Source: CAD feature listing. Evaluate the final solid. Frame: model axes, mm. A direction names the side the tool comes from. Give positions to 0.01 mm unless a question says otherwise; leave off trailing zeros. Loops run counter-clockwise (first coordinate to the right, second up) from the corner with the lowest first, then second, coordinate; pieces in that order, holes last. Notation, with made-up numbers: M 28,75.25 L 84,75.25 A30 ccw 84,110.25 Z; hole C -6.75,59 d11. An arc over 180 degrees is marked long. Write item = value, one per line.
from build123d import *

# Parameters (mm, degrees)
F1_DEPTH = 10
F2_R     = 1
F3_R     = 3
F4_R     = 0.33333


with BuildPart() as f1:
    # F0 (on Front) → F1 (new body)
    with BuildSketch(Plane.XZ):
        with BuildLine():
            Line((0, 0), (3.6, 0))
            Line((3.6, 0), (3.6, 3))
            Line((3.6, 3), (1.8, 3))
            Line((1.8, 3), (1.8, 11.7))
            Line((1.8, 11.7), (5.8, 11.7))
            Line((5.8, 11.7), (5.8, 8.7))
            Line((5.8, 8.7), (6.6518087818, 8.6985993288))
            ThreePointArc((6.6518087818, 8.6985993288), (7.4284566976, 8.3757785113), (7.75, 7.598600816))
            Line((7.75, 7.598600816), (9.25, 7.598600816))
            Line((9.25, 7.598600816), (7, 13.5))
            Line((7, 13.5), (0, 13.5))
            Line((0, 13.5), (0, 0))
        make_face()
        with BuildLine():
            ThreePointArc((6.4457045279, 5.2862485499), (8.0654097754, 6.1785827272), (9.25, 7.598600816))
            Line((9.25, 7.598600816), (7.75, 7.598600816))
            ThreePointArc((7.75, 7.598600816), (7.4278174593, 6.8207833567), (6.65, 6.498600816))
            Line((6.65, 6.498600816), (5.8, 6.498600816))
            Line((5.8, 6.498600816), (5.8, 5.2862485499))
            Line((5.8, 5.2862485499), (6.4457045279, 5.2862485499))
        make_face()
    extrude(amount=F1_DEPTH)

    # F2
    f2_edges = [f1.edges().sort_by_distance(p)[0] for p in [
        (0, -5, 13.5),
        (7, -5, 13.5),
        (6.445705, -5, 5.286249),
        (9.25, -5, 7.598601),
    ]]
    fillet(f2_edges, radius=F2_R)

    # F3
    f3_edges = [f1.edges().sort_by_distance(p)[0] for p in [
        (0, -5, 0),
    ]]
    fillet(f3_edges, radius=F3_R)

    # F4
    f4_edges = [f1.edges().sort_by_distance(p)[0] for p in [
        (5.8, -5, 11.7),
        (5.8, -5, 5.286249),
        (5.8, -5, 6.498601),
        (1.8, -5, 3),
        (1.8, -5, 11.7),
    ]]
    fillet(f4_edges, radius=F4_R)


solid = f1.part
1. First-contact query: pin 1 Ø0.9 at (y, z) = (-4.5, 1.5) entering from +X; pin 2 Ø3 at (x, y) = (2.5, -7.5) entering from -Z; pin 3 Ø2 at (x, y) = (8, -2.5) entering from +Z. Flat tips, straight axial feed; report the tip coordinate or a pass-through.
Derived:
pin_1 = 3.6
pin_2 = 0
pin_3 = 13.22
2. Material intervals for probe 1 along Z at (x, y) = (3.25, -1.5); probe 2 along Z at (x, y) = (7, -0.75); probe 3 along Z at (x, y) = (4, -7.25), sorted ascending. Write a range as from..to.
Derived:
probe_1 = 0..3, 11.7..13.5
probe_2 = 5.51..6.56, 8.64..13.22
probe_3 = 11.7..13.5
3. Pull-direction query (Z, two-part tool) for faces 1 (the flat face through (1.8, -5, 7)), 2 (the cylindrical face through (7.9, -4.93, 6.05)), 3 (the flat face through (4, -5, 11.7)), 4 (the flat face through (4, -5, 13.5)); classes: +Z half, -Z half, draft (parallel to the pull), parting line (faces both ways), or undercut.
Derived:
face_1 = undercut
face_2 = -Z half
face_3 = undercut
face_4 = +Z half
4. Cut plane C-C, the plane y = -1.25. Return the cut outline in (x, z), then the cut area to 3 significant figures.
Derived:
outline = M 0,3 A3 ccw 3,0 L 3.6,0 L 3.6,3 L 2.13,3 A0.33 cw 1.8,3.33 L 1.8,11.37 A0.33 cw 2.13,11.7 L 5.47,11.7 A0.33 cw 5.8,11.37 L 5.8,8.7 L 6.65,8.7 A1.1 cw 6.65,6.5 L 6.13,6.5 A0.33 ccw 5.8,6.17 L 5.8,5.62 A0.33 ccw 6.13,5.29 L 6.28,5.29 A1 ccw 6.62,5.35 A5 ccw 8.95,7.13 A1 ccw 9.07,8.07 L 7.25,12.86 A1 ccw 6.31,13.5 L 1,13.5 A1 ccw 0,12.5 Z
area = 50.2 mm²
5. Cut plane B-B, the plane z = 6. Return the cut outline in (x, y).
Derived:
outline = M 0,-10 L 1.8,-10 L 1.8,0 L 0,0 Z; M 5.8,-10 L 7.84,-10 L 7.84,0 L 5.8,0 Z
6. Cut plane D-D, the plane x = 4.75. Return the cut outline in (y, z).
Derived:
outline = M -10,11.7 L 0,11.7 L 0,13.5 L -10,13.5 Z
7. Cut plane A-A, the plane x = 2.75. Return the cut outline in (y, z), then the cut area to 3 significant figures.
Derived:
outline = M -10,0.01 L 0,0.01 L 0,3 L -10,3 Z; M -10,11.7 L 0,11.7 L 0,13.5 L -10,13.5 Z
area = 47.9 mm²
8. Reachability of faces 5 (the flat face through (1, 0, 8)), 6 (the flat face through (3, -5, 3)), 7 (the flat face through (0, -5, 8)), 8 (the flat face through (3.6, -5, 1)), 9 (the flat face through (5.8, -5, 10)) from +Z, -Z, +X, -X, +Y, -Y: full face, straight path, thin tool, end or side. Return the list, or none.
Derived:
face_5 = +Z, -Z, +X, -X, +Y
face_6 = +X, +Y, -Y
face_7 = +Z, -Z, -X, +Y, -Y
face_8 = -Z, +X, +Y, -Y
face_9 = -Z, +Y, -Y
